Build history of the part. All positions in model axes, mm. Face numbers are marked on the shaded views. A direction names the side the tool comes from. Round coordinates to 2 decimals unless told otherwise and drop trailing zeros. Write each loop counter-clockwise with the first axis right and the second up, starting at its lowest first coordinate (ties: lowest second). Pieces come first, ordered by that corner, then holes. Notation, with made-up numbers: (74.25, 46.25) - (92.25, 46.25) arc R25 ccw to (92.25, 70.25) - close; hole circle Ø6 at (41.5, 77.25). An arc over 180 degrees is marked (long way). One line per question, with ' | ' between items.
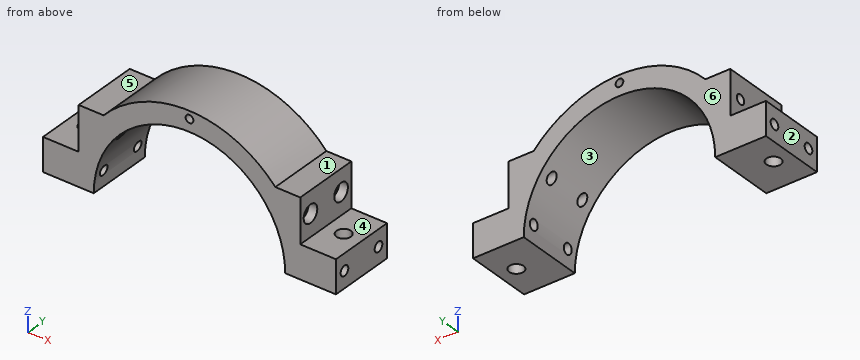
from build123d import *

# Parameters (mm, degrees)
BOSS_EXTRUDE1_DEPTH            = 15
SKETCH2_R                      = 3.25
CUT_EXTRUDE1_DEPTH             = 78.406027705
SKETCH3_R                      = 2.25
CUT_EXTRUDE2_DEPTH             = 144.078946739
CUT_EXTRUDE3_DEPTH             = 90.494095583
CUT_EXTRUDE3_DEPTH_BACK        = 90.494095583
SKETCH4_R                      = 1.75
BOSS_EXTRUDE2_DEPTH            = 30
CBORE_FOR_M4_SHCS1_D           = 4.3
CBORE_FOR_M4_SHCS1_DEPTH       = 100.101198794
CBORE_FOR_M4_SHCS1_CBORE_D     = 8
CBORE_FOR_M4_SHCS1_CBORE_DEPTH = 4
CBORE_FOR_M4_SHCS1_TIP         = 1.291850331


with BuildPart() as part:
    # Sketch1 → Boss-Extrude1 (new, symmetric)
    with BuildSketch(Plane(origin=(0, 0, 0), x_dir=(1, 0, 0), z_dir=(0, 1, 0))):
        with BuildLine():
            Line((-43.25, 0), (-66.175, 0))
            Line((-66.175, 0), (-66.175, -15))
            Line((-66.175, -15), (-50.050599397, -15))
            ThreePointArc((-50.050599397, -15), (0, -52.25), (50.050599397, -15))
            Line((50.050599397, -15), (66.175, -15))
            Line((66.175, -15), (66.175, 0))
            Line((66.175, 0), (43.25, 0))
            ThreePointArc((43.25, 0), (0, -43.25), (-43.25, 0))
        make_face()
    extrude(amount=BOSS_EXTRUDE1_DEPTH, both=True)

    # Sketch2 → Cut-Extrude1 (cut, through all)
    with BuildSketch(Plane.XY.offset(15)):
        with Locations((-58.112799699, 0)):
            Circle(SKETCH2_R)
        with Locations((58.112799699, 0)):
            Circle(SKETCH2_R)
    extrude(amount=-CUT_EXTRUDE1_DEPTH, mode=Mode.SUBTRACT)

    # Sketch3 → Cut-Extrude2 (cut, through all)
    with BuildSketch(Plane.ZY.offset(66.175)):
        with Locations((7.5, -10)):
            Circle(SKETCH3_R)
        with Locations((7.5, 10)):
            Circle(SKETCH3_R)
    extrude(amount=-CUT_EXTRUDE2_DEPTH, mode=Mode.SUBTRACT)

    # Sketch4 → Cut-Extrude3 (cut, two sides: drawn at the far end of the back side and taken through both)
    with BuildSketch(Plane(origin=(0, 15, 0), x_dir=(1, 0, 0), z_dir=(0, 1, 0)).offset(-CUT_EXTRUDE3_DEPTH_BACK)):
        with Locations(Location((0, -48.75, 0), (0, 0, 270))):
            Circle(SKETCH4_R)
    extrude(amount=CUT_EXTRUDE3_DEPTH + CUT_EXTRUDE3_DEPTH_BACK, mode=Mode.SUBTRACT)

    # Sketch5 → Boss-Extrude2 (add)
    with BuildSketch(Plane(origin=(0, 15, 0), x_dir=(1, 0, 0), z_dir=(0, 1, 0))):
        with BuildLine():
            Line((-50.050599397, -15), (-50.050599397, -35))
            Line((-50.050599397, -35), (-38.795135004, -35))
            ThreePointArc((-38.795135004, -35), (-45.534504832, -25.625599889), (-50.050599397, -15))
        make_face()
    boss_extrude2 = extrude(amount=-BOSS_EXTRUDE2_DEPTH)

    # Mirror1: Boss-Extrude2 across plane
    add(boss_extrude2.mirror(Plane.ZY))

    # CBORE for M4 SHCS1
    with Locations(Plane(origin=(50.050599397, 54.222001278, 632.558854999), x_dir=(0, -0.9379679207103062, -0.3467220496570483), z_dir=(1, 0, 0))):
        with Locations((253.070838002, 554.191250959), (269.954260575, 547.950254066)):
            CounterBoreHole(CBORE_FOR_M4_SHCS1_D / 2, CBORE_FOR_M4_SHCS1_CBORE_D / 2, CBORE_FOR_M4_SHCS1_CBORE_DEPTH, depth=CBORE_FOR_M4_SHCS1_DEPTH)
            with Locations((0, 0, -(CBORE_FOR_M4_SHCS1_DEPTH + CBORE_FOR_M4_SHCS1_TIP / 2))):  # 118° drill point
                Cone(0, CBORE_FOR_M4_SHCS1_D / 2, CBORE_FOR_M4_SHCS1_TIP, mode=Mode.SUBTRACT)


solid = part.part
Q1. Drill centre lines: L1, parallel to Y at x = 47, z = 25; L2, parallel to Y at x = -49, z = 7; L3, parallel to Z at x = -56, y = -10. Where is each one in solid material? Low to high. Write a range as from..to.
Found:
L1: -15..-13, -5..5, 13..15 | L2: -15..-12.19, -7.81..7.81, 12.19..15 | L3: 0..5.25, 9.75..15
Q2. Saw through at B-B, the plane z = 38.5. List the corners of the cut face in (x, y).
Found:
outline: (-35.32, -15) - (-19.71, -15) - (-19.71, 15) - (-35.32, 15) - close; (19.71, -15) - (35.32, -15) - (35.32, 15) - (19.71, 15) - close
Q3. Saw through at D-D, the plane x = -15. List the corners of the cut face in (y, z).
Found:
outline: (-15, 40.57) - (15, 40.57) - (15, 50.05) - (-15, 50.05) - close
Q4. Pull direction X, two halves, no side cores. Call the marked faces 1, 2 and 3: +X half, -X half, draft (parallel to the pull), parting line (faces both ways), or undercut.
Found:
face 1: draft | face 2: -X half | face 3: undercut
Q5. Saw through at A-A, the plane z = 12.5. List the corners of the cut face in (x, y) (3 decimals), then the cut area to 3 significant figures.
Found:
outline: (-66.175, -15) - (-41.404, -15) - (-41.404, 15) - (-66.175, 15) - close; (41.404, -15) - (66.175, -15) - (66.175, 15) - (41.404, 15) - close; hole circle Ø6.5 at (-58.113, 0); hole circle Ø6.5 at (58.113, 0) | area: 1,420 mm^2
Q6. Which spindle directions (+Z, -Z, +X, -X, +Y, -Y) get a long thin tool onto all of the face, cutting with end or side? Do the marked faces 4, 5 and 6. Say none if no direction does.
Found:
face 4: +Z, +X, +Y, -Y | face 5: +Z, -X, +Y, -Y | face 6: +Z, -Z, +X, -X, +Y
Q7. Saw through at C-C, the plane z = 3.5. List the corners of the cut face in (x, y) (3 decimals).
Found:
outline: (-66.175, -15) - (-43.108, -15) - (-43.108, 15) - (-66.175, 15) - close; (43.108, -15) - (66.175, -15) - (66.175, 15) - (43.108, 15) - close; hole circle Ø6.5 at (-58.113, 0); hole circle Ø6.5 at (58.113, 0)
Q8. Drop flat-ended pins along their axis: pin 1 (7 mm diameter, centred on y = 9, z = 25, fed in from +X); pin 2 (12 mm diameter, centred on x = -1.5, y = 2.5, fed in from -Z); pin 3 (7.5 mm diameter, centred on x = -58.11, y = 0, fed in from +Z). Give the stop position or say it passes through.
Found:
pin 1: x = 46.05 | pin 2: z = 42.59 | pin 3: z = 15
